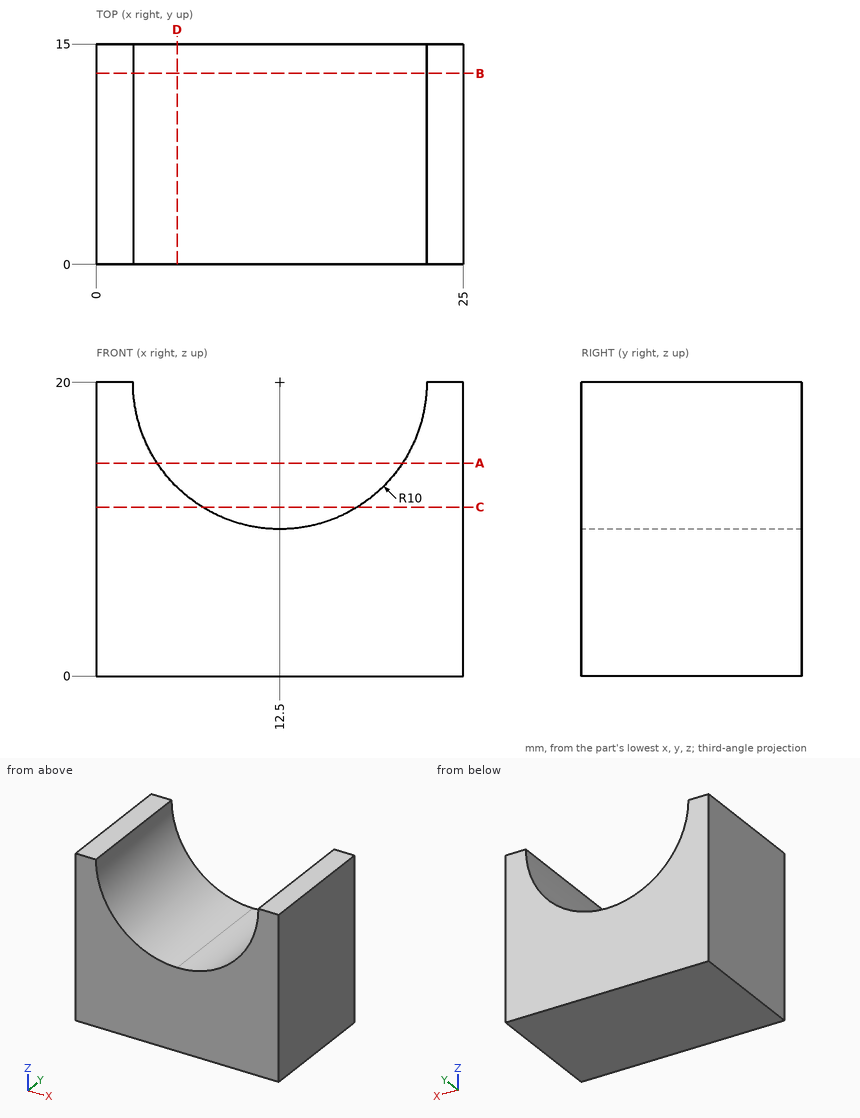
Can you work these out from the drawing? Everything is in mm from the part's minimum corner. Coordinates: 2 decimals unless noted, no trailing zeros. Order: outer loops, then holes, each group sorted by start corner. A loop starts at its lowest first (then second) coordinate and runs counter-clockwise, first axis right, second up. Notation, with made-up numbers: (-27.75, 33) -> (-8.75, 33) arc R16 cw to (-8.75, 58) -> close; hole circle Ø7 at (82.5, -11). An arc over 180 degrees is marked (long way). Return JSON: item names as keys, results as strings.
1) If I drill on probe 1 along X at (y, z) = (8.5, 16); probe 2 along X at (y, z) = (4.5, 18.75); probe 3 along Z at (x, y) = (6, 1.5), over which ranges is the centre line in solid material (lowest first)?
Conclusion:
{"probe 1": "x = 0 to 3.33, 21.67 to 25", "probe 2": "x = 0 to 2.58, 22.42 to 25", "probe 3": "z = 0 to 12.4"}
2) If we section it at A-A on z = 14.5: List the corners of the cut face in (x, y) for me, plus the area to 3 significant figures.
Conclusion:
{"outline": "(0, 0) -> (4.15, 0) -> (4.15, 15) -> (0, 15) -> close; (20.85, 0) -> (25, 0) -> (25, 15) -> (20.85, 15) -> close", "area": "124 mm²"}
3) If we section it at C-C on z = 11.5: List the corners of the cut face in (x, y) for me, plus the area to 3 significant figures.
Conclusion:
{"outline": "(0, 0) -> (7.23, 0) -> (7.23, 15) -> (0, 15) -> close; (17.77, 0) -> (25, 0) -> (25, 15) -> (17.77, 15) -> close", "area": "217 mm²"}
4) If we section it at D-D on x = 5.5: List the corners of the cut face in (y, z) for me.
Conclusion:
{"outline": "(0, 0) -> (15, 0) -> (15, 12.86) -> (0, 12.86) -> close"}
5) If we section it at B-B on y = 13: List the corners of the cut face in (x, z) for me.
Conclusion:
{"outline": "(0, 0) -> (25, 0) -> (25, 20) -> (22.5, 20) arc R10 cw to (12.5, 10) arc R10 cw to (2.5, 20) -> (0, 20) -> close"}
6) I'm going to push flat-ended pins straight in: P1, Ø6, axis at x = 8, y = 13, coming from the -Z side; P2, Ø4, axis at x = 9, y = 12, coming from the +Z side. Where does each tip first touch, or does it pass through?
Conclusion:
{"P1": "stops at z = 0", "P2": "stops at z = 11.65"}
